Autodesk Inventor part; units mm, degrees
ref_plane "YZ Plane" through (0, 0, 0) normal (1, 0, 0) x (0, 1, 0)
ref_plane "XZ Plane" through (0, 0, 0) normal (0, 1, 0) x (-1, 0, 0)
ref_plane "XY Plane" through (0, 0, 0) normal (0, 0, 1) x (1, 0, 0)
sketch "Sketch1" plane through (0, 0, 0) normal (0, 0, 1) x (1, 0, 0)
  circle A0 centre (0, 0) radius 2.4
  dimension "d0" = 4.8
extrude "Extrusion1" add sketch "Sketch1" along normal blind 6
sketch "Sketch2" plane through (0, 0, 6) normal (0, 0, 1) x (1, 0, 0)
  point P0 (0, 0)
  point P1 (0, 0)
hole "Hole1" at (0, 0, 6) direction (0, 0, -1) diameter 2.459 end through all
chamfer "Chamfer1" distance 0.2 angle 45 2 edges at (-2.4, 0, 6) (-2.4, 0, 0)
chamfer "Chamfer2" distance 0.1 angle 45 2 edges at (0, 1.2295, 6) (0, 1.2295, 0)
thread "Thread2"
sketch "Sketch4" plane through (0, 0, 0) normal (0, 1, 0) x (-1, 0, 0)
  line L0 (-0.5, 0) -> (0.5, 0)
  line L1 (0.5, 0) -> (0.5, 2)
  line L2 (0.5, 2) -> (-0.5, 2)
  line L3 (-0.5, 2) -> (-0.5, 0)
  point P0 (0, 0)
  dimension "d22" = 1
  dimension "d23" = 0.5
  dimension "d24" = 2
extrude "Extrusion2" cut sketch "Sketch4" along normal mid plane 6
properties part number "XGEN_M3_draadbus_4x6mm"
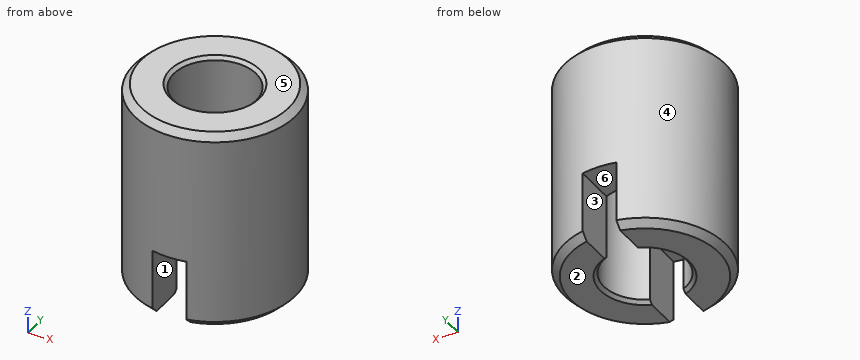
Check sheet for the modelled part. Datum: model origin and axes. Units: mm. Face numbers are marked on the shaded views. A direction names the side the tool comes from. Round coordinates to 2 decimals unless told otherwise and drop trailing zeros. Order: outer loops, then holes, each group sorted by start corner. A loop starts at its lowest first (then second) coordinate and runs counter-clockwise, first axis right, second up.
(1) Cross-section at C-C, the plane z = 0.6. Enter the section's corners in (x, y), and give its area (3 significant figures).
(2) Go/stop test with flat-tipped pins: P1, Ø0.8, axis at x = 0, y = 1.5, coming from the -Z side; P2, Ø0.6, axis at y = 2, z = 0.5, coming from the +X side; P3, Ø1, axis at y = -1.5, z = 1.5, coming from the +X side; P4, Ø1.5, axis at x = -0.5, z = 2, coming from the +Y side. Record where each tip stops, or that it passes through.
(3) Cross-section at B-B, the plane y = 0. Enter the section's corners in (x, z), and give its area (3 significant figures).
(4) Draft check along X on the marked faces 1, 2, 3 and 4. Enter one of: pulls with the +X half, pulls with the -X half, needs draft (parallel to the pull), parting line crosses it, or undercut.
(5) Access from +Z, -Z, +X, -X, +Y, -Y to the whole of each face (thin tool, end or side, straight path). Record for the marked faces 5 and 6.
(6) Cross-section at A-A, the plane x = 0. Enter the section's corners in (y, z), and give its area (3 significant figures).
(7) Scan lines: probe 1 along X at (y, z) = (0, 4.55); probe 2 along Z at (x, y) = (-0.3, 1.75). Record each from-to range of solid material in increasing order.
Check sheet entries:
1. outline: (-0.5, -2.35) - (-0.5, -1.12) arc R1.23 cw to (-0.5, 1.12) - (-0.5, 2.35) arc R2.4 ccw to start; (0.5, -2.35) arc R2.4 ccw to (0.5, 2.35) - (0.5, 1.12) arc R1.23 cw to (0.5, -1.12) - close
1. area: 11.0 mm2
2. P1: stops at z = 2
2. P2: stops at x = 1.69
2. P3: stops at x = 2.18
2. P4: stops at y = 2.4
3. outline: (-2.4, 0.2) - (-2.2, 0) - (-1.33, 0) - (-1.23, 0.1) - (-1.23, 5.9) - (-1.33, 6) - (-2.2, 6) - (-2.4, 5.8) - close; (1.23, 0.1) - (1.33, 0) - (2.2, 0) - (2.4, 0.2) - (2.4, 5.8) - (2.2, 6) - (1.33, 6) - (1.23, 5.9) - close
3. area: 13.9 mm2
4. face 1: undercut
4. face 2: needs draft
4. face 3: undercut
4. face 4: parting line crosses it
5. face 5: +Z, +X, -X, +Y, -Y
5. face 6: -Z, +Y, -Y
6. outline: (-2.4, 2) - (-1.23, 2) - (-1.23, 5.9) - (-1.33, 6) - (-2.2, 6) - (-2.4, 5.8) - close; (1.23, 2) - (2.4, 2) - (2.4, 5.8) - (2.2, 6) - (1.33, 6) - (1.23, 5.9) - close
6. area: 9.31 mm2
7. probe 1: x = -2.4 to -1.23, 1.23 to 2.4
7. probe 2: z = 2 to 6
